Source: CAD feature listing. Evaluate the final solid. Frame: model axes, mm. A direction names the side the tool comes from. Give positions to 0.01 mm unless a question says otherwise; leave off trailing zeros. Loops run counter-clockwise (first coordinate to the right, second up) from the corner with the lowest first, then second, coordinate; pieces in that order, holes last. Notation, with made-up numbers: (35, 13.5) - (91, 13.5) arc R4 ccw to (91, 18.5) - close; hole circle Ø6 at (-34.75, 89). An arc over 180 degrees is marked (long way). Put each result on its own line as item: value.
Autodesk Inventor part; units mm, degrees
ref_plane "YZ Plane" through (0, 0, 0) normal (1, 0, 0) x (0, 1, 0)
ref_plane "XZ Plane" through (0, 0, 0) normal (0, 1, 0) x (-1, 0, 0)
ref_plane "XY Plane" through (0, 0, 0) normal (0, 0, 1) x (1, 0, 0)
ref_plane "Work Plane1" through (0, 0, 0) normal (0, 0, 1) x (1, 0, 0)
sketch "Sketch1" plane through (0, 0, 0) normal (0, 0, 1) x (1, 0, 0)
  line L0 (-295.275, -1057.275) -> (454.025, -1057.275)
  line L1 (454.025, -1057.275) -> (454.025, 962.025)
  circle A0 centre (384.175, -28.575) radius 31.4325
  line L2 (454.025, 962.025) -> (-295.275, 962.025)
  line L3 (-295.275, 962.025) -> (-295.275, -1057.275)
  line L4 (462.153, 970.153) -> (462.153, -1065.403)
  line L5 (462.153, -1065.403) -> (-303.403, -1065.403)
  line L6 (-303.403, -1065.403) -> (-303.403, 970.153)
  line L7 (-303.403, 970.153) -> (462.153, 970.153)
  line L8 (500.253, -1103.503) -> (500.253, 1008.253)
  line L9 (500.253, 1008.253) -> (-341.503, 1008.253)
  line L10 (-341.503, 1008.253) -> (-341.503, -1103.503)
  line L11 (-341.503, -1103.503) -> (500.253, -1103.503)
  point P0 (-454.025, -1057.275)
  point P1 (454.025, 1057.275)
  point P2 (-454.025, 1057.275)
  point P3 (-454.025, 933.45)
  point P4 (-454.025, 819.15)
  point P5 (-454.025, 114.3)
  point P6 (-454.025, 0)
  point P7 (-454.025, -704.85)
  point P8 (-454.025, -819.15)
  dimension "d17" = 8.128
  dimension "d18" = 38.1
extrude "Extrusion1" add sketch "Sketch1" along normal blind 95.25 and the other way blind 44.45 contours L11 L10 L9 L8
sketch "Sketch2" plane through (-341.503, 1008.253, 95.25) normal (0, 1, 0) x (1, 0, 0)
  circle A0 centre (147.6845, 40.534) radius 3.175
  point P0 (341.503, 95.25)
  dimension "d19" = 6.35
extrude "Extrusion2" cut sketch "Sketch2" against normal blind 95.25
properties part number "DoorFrame"
1) Material intervals for line 1 along Y through (x, z) = (280.5, 0); line 2 along X through (y, z) = (-110, -23), sorted ascending. Write a range as [from, to].
Check result:
line 1: [-1103.5, -1065.4], [970.15, 1008.25]
line 2: [-341.5, -303.4], [462.15, 500.25]
2) Mould query, pull axis Y, two halves, no side actions, for faces 1 (the flat face through (462.153, -33, 24)), 2 (the flat face through (85, 1008.253, 24)), 3 (the flat face through (500.253, -62, 24)). Classes: pulls with the +Y half, pulls with the -Y half, needs draft (parallel to the pull), parting line crosses it, or undercut.
Check result:
face 1: undercut
face 2: pulls with the +Y half
face 3: needs draft
3) Access query for faces 4 (the flat face through (73, -1103.503, 24)), 5 (the flat face through (74, 970.153, 24)). Directions: +Z, -Z, +X, -X, +Y, -Y. A direction counts if a zero-diameter tool reaches every point of the face in a straight line with its end or side. Return the directions, or none.
Check result:
face 4: +Z, -Z, +X, -X, -Y
face 5: +Z, -Z
4) Section query B-B, the plane y = 274.5. Output: boundary loops of the cut face in (x, z), plus the area to 3 significant figures.
Check result:
outline: (-341.5, -44.45) - (-303.4, -44.45) - (-303.4, 95.25) - (-341.5, 95.25) - close; (462.15, -44.45) - (500.25, -44.45) - (500.25, 95.25) - (462.15, 95.25) - close
area: 10,600 mm²
5) Section query C-C, the plane z = -11. Output: boundary loops of the cut face in (x, y).
Check result:
outline: (-341.5, -1103.5) - (500.25, -1103.5) - (500.25, 1008.25) - (-341.5, 1008.25) - close; hole (-303.4, -1065.4) - (462.15, -1065.4) - (462.15, 970.15) - (-303.4, 970.15) - close
6) Section query A-A, the plane x = -157. Output: boundary loops of the cut face in (y, z).
Check result:
outline: (-1103.5, -44.45) - (-1065.4, -44.45) - (-1065.4, 95.25) - (-1103.5, 95.25) - close; (970.15, -44.45) - (1008.25, -44.45) - (1008.25, 95.25) - (970.15, 95.25) - close
